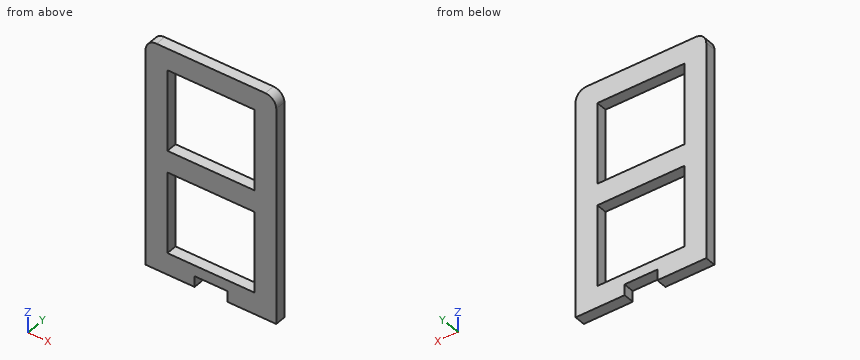
```python
from build123d import *

# Parameters (mm, degrees)
SKETCH1_W           = 60
SKETCH1_H           = 5
BOSS_EXTRUDE1_DEPTH = 105
SKETCH2_W           = 40
SKETCH2_H           = 37.5
CUT_EXTRUDE1_DEPTH  = 105
FILLET1_R           = 5
SKETCH4_W           = 15
SKETCH4_H           = 10
CUT_EXTRUDE3_DEPTH  = 10


with BuildPart() as part:
    # Sketch1 → Boss-Extrude1 (new body)
    with BuildSketch(Plane.XY):
        Rectangle(SKETCH1_W, SKETCH1_H)
    extrude(amount=BOSS_EXTRUDE1_DEPTH)

    # Sketch2 → Cut-Extrude1 (cut)
    with BuildSketch(Plane.XZ.offset(2.5)):
        with Locations((0, 28.75)):
            Rectangle(SKETCH2_W, SKETCH2_H)
        with Locations((0, 76.25)):
            Rectangle(SKETCH2_W, SKETCH2_H)
    extrude(amount=-CUT_EXTRUDE1_DEPTH, mode=Mode.SUBTRACT)

    # Fillet1
    fillet1_edges = [part.edges().sort_by_distance(p)[0] for p in [
        (-30, 0, 105),
        (30, 0, 105),
    ]]
    fillet(fillet1_edges, radius=FILLET1_R)

    # Sketch4 → Cut-Extrude3 (cut)
    with BuildSketch(Plane.XZ.offset(2.5)):
        Rectangle(SKETCH4_W, SKETCH4_H)
    extrude(amount=-CUT_EXTRUDE3_DEPTH, mode=Mode.SUBTRACT)


solid = part.part
```
For this review, take the finished solid that the model builds, in its own axes (mm). Round coordinates to 2 decimals unless told otherwise and drop trailing zeros. Write each loop counter-clockwise with the first axis right and the second up, starting at its lowest first coordinate (ties: lowest second). Pieces come first, ordered by that corner, then holes. Notation, with made-up numbers: (76, 10) - (112, 10) arc R23 ccw to (112, 39) - close; hole circle Ø9 at (44.25, -4.5). An arc over 180 degrees is marked (long way). Use CSV: the item, a comma, the result in double quotes.
1) Add section D-D on x = 0. Write out the cut boundary in (y, z).
Conclusion:
outline,"(-2.5, 5) - (2.5, 5) - (2.5, 10) - (-2.5, 10) - close; (-2.5, 47.5) - (2.5, 47.5) - (2.5, 57.5) - (-2.5, 57.5) - close; (-2.5, 95) - (2.5, 95) - (2.5, 105) - (-2.5, 105) - close"
2) Clearance check with a flat-ended pin moving along its axis: pin 1 Ø2.5 at (x, y) = (3, 1) entering from -Z. State where the tip first meets the part, or that it passes through.
Conclusion:
pin 1,"stops at z = 5"
3) Wall thickness on line 1 along Z through (x, y) = (17, 0); line 2 along Z through (x, y) = (5, 0.3); line 3 along X through (y, z) = (-2, 89): over which ranges is each line inside the solid? List them lowest first. Write a range as from..to.
Conclusion:
line 1,"z = 0..10, 47.5..57.5, 95..105"
line 2,"z = 5..10, 47.5..57.5, 95..105"
line 3,"x = -30..-20, 20..30"
4) Add section C-C on y = -0.2. Write out the cut boundary in (x, z).
Conclusion:
outline,"(-30, 0) - (-7.5, 0) - (-7.5, 5) - (7.5, 5) - (7.5, 0) - (30, 0) - (30, 100) arc R5 ccw to (25, 105) - (-25, 105) arc R5 ccw to (-30, 100) - close; hole (-20, 10) - (20, 10) - (20, 47.5) - (-20, 47.5) - close; hole (-20, 57.5) - (20, 57.5) - (20, 95) - (-20, 95) - close"
5) Add section B-B on x = 18. Write out the cut boundary in (y, z).
Conclusion:
outline,"(-2.5, 0) - (2.5, 0) - (2.5, 10) - (-2.5, 10) - close; (-2.5, 47.5) - (2.5, 47.5) - (2.5, 57.5) - (-2.5, 57.5) - close; (-2.5, 95) - (2.5, 95) - (2.5, 105) - (-2.5, 105) - close"
6) Add section A-A on z = 45.5. Write out the cut boundary in (x, y), and give its area (3 significant figures).
Conclusion:
outline,"(-30, -2.5) - (-20, -2.5) - (-20, 2.5) - (-30, 2.5) - close; (20, -2.5) - (30, -2.5) - (30, 2.5) - (20, 2.5) - close"
area,"100 mm^2"
